from build123d import *

# Parameters (mm, degrees)
SKETCH2_W           = 53.1368
SKETCH2_H           = 28.9814
SKETCH2_W_2         = 5.3848
SKETCH2_H_2         = 3.1242
BOSS_EXTRUDE1_DEPTH = 12.3952
SKETCH3_R           = 4.4831
BOSS_EXTRUDE2_DEPTH = 33.4772
SKETCH5_W           = 3.937
SKETCH5_H           = 3.937
BOSS_EXTRUDE3_DEPTH = 3.048


with BuildPart() as part:
    # Sketch2 → Boss-Extrude1 (new body)
    with BuildSketch(Plane(origin=(0, 0, 0), x_dir=(1, 0, 0), z_dir=(0, 1, 0))):
        Rectangle(SKETCH2_W, SKETCH2_H)
        Polygon((26.5684, -14.4907), (25.2984, -14.4907), (25.2984, -17.6149), (26.5684, -16.3449), align=None)
        with Locations((22.606, -16.0528)):
            Rectangle(SKETCH2_W_2, SKETCH2_H_2)
        Polygon((19.9136, -14.4907), (16.7894, -14.4907), (19.9136, -17.6149), align=None)
        Polygon((-26.5684, -16.3449), (-25.2984, -17.6149), (-25.2984, -14.4907), (-26.5684, -14.4907), align=None)
        with Locations((-22.606, -16.0528)):
            Rectangle(SKETCH2_W_2, SKETCH2_H_2)
        Polygon((-19.9136, -14.4907), (-19.9136, -17.6149), (-16.7894, -14.4907), align=None)
    extrude(amount=BOSS_EXTRUDE1_DEPTH)

    # Sketch3 → Boss-Extrude2 (add)
    with BuildSketch(Plane(origin=(0, 0, -14.4907), x_dir=(-1, 0, 0), z_dir=(0, 0, -1))):
        with Locations(Location((18.6309, 7.9121, 0), (0, 0, 90))):
            Circle(SKETCH3_R)
    extrude(amount=BOSS_EXTRUDE2_DEPTH)

    # Sketch5 → Boss-Extrude3 (add)
    with BuildSketch(Plane(origin=(0, 12.3952, 0), x_dir=(1, 0, 0), z_dir=(0, 1, 0))):
        with Locations((-8.3185, 8.6106)):
            Rectangle(SKETCH5_W, SKETCH5_H)
    extrude(amount=BOSS_EXTRUDE3_DEPTH)


solid = part.part
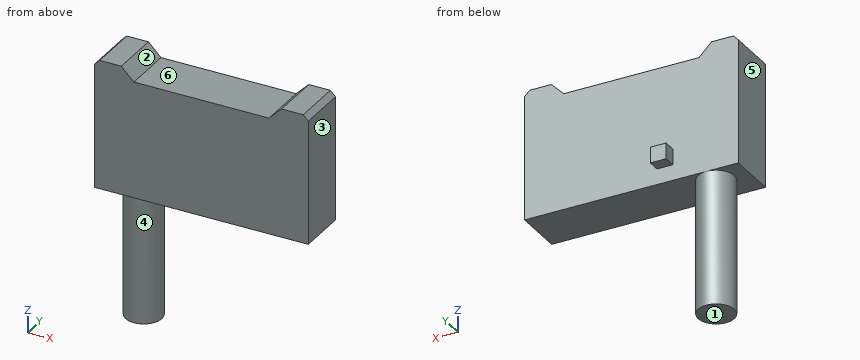
Check sheet for the modelled part. Datum: model origin and axes. Units: mm. Face numbers are marked on the shaded views. A direction names the side the tool comes from. Give positions to 0.01 mm unless a question says otherwise; leave off trailing zeros. Loops run counter-clockwise (first coordinate to the right, second up) from the corner with the lowest first, then second, coordinate; pieces in that order, holes last. Notation, with made-up numbers: M 87.25,-16.5 L 97.25,-16.5 A13 ccw 97.25,-10.5 Z; hole C 5.5,11 d8. An arc over 180 degrees is marked long. Use a Markdown table: item, result. Add a question column.
Q1. Tool access check on the marked faces 5 and 6. Record the directions out of +Z, -Z, +X, -X, +Y, -Y that give a thin tool (end or side, any length) a straight path to the whole face; none if there is none.
Q2. Sectioned sample at D-D, the plane x = 7. Record the cut outline in (y, z).
Q3. Sectioned sample at B-B, the plane x = -15.5. Record the cut outline in (y, z), then the cut area to 3 significant figures.
Q4. Sectioned sample at A-A, the plane y = 7.5. Record the cut outline in (x, z), then the cut area to 3 significant figures.
Q5. Scan lines: line 1 along X through (y, z) = (13, -8.5); line 2 along Z through (x, y) = (10.5, 10.25); line 3 along Z through (x, y) = (-9.5, 14.25). Record each from-to range of solid material in increasing order. Write a range as [from, to].
Q6. Mould release check, pull along X, two halves, no side actions. Record for the marked faces 1, 2, 3 and 4: pulls with the +X half, pulls with the -X half, needs draft (parallel to the pull), parting line crosses it, or undercut.
Q7. Go/stop test with flat-tipped pins: pin 1 (3.5 mm diameter, centred on x = -9, y = 13.5, fed in from +Z); pin 2 (0.9 mm diameter, centred on y = 14, z = -8, fed in from -X); pin 3 (6 mm diameter, centred on x = -11, y = 6.5, fed in from -Z). Record where each tip stops, or that it passes through.
Q8. Sectioned sample at C-C, the plane z = 0.5. Record the cut outline in (x, y), then the cut area to 3 significant figures.
Verdict:
| question | item | result |
|---|---|---|
| 1 | face 5 | +Z, -Z, -X, +Y, -Y |
| 1 | face 6 | +Z, +Y, -Y |
| 2 | outline | M 0,-14.49 L 12.4,-14.49 L 12.4,14.49 L 0,14.49 Z |
| 3 | outline | M 0,-14.49 L 4.7,-14.49 L 4.7,-47.97 L 11.12,-47.97 L 11.12,-14.49 L 12.4,-14.49 L 12.4,14.49 L 0,14.49 Z |
| 3 | area | 574 mm^2 |
| 4 | outline | M -26.57,-14.49 L -23.1,-14.49 L -23.1,-47.97 L -14.17,-47.97 L -14.17,-14.49 L 26.57,-14.49 L 26.57,16.34 L 25.3,17.61 L 19.91,17.61 L 16.79,14.49 L -16.79,14.49 L -19.91,17.61 L -25.3,17.61 L -26.57,16.34 Z |
| 4 | area | 1,890 mm^2 |
| 5 | line 1 | [-10.29, -6.35] |
| 5 | line 2 | [-14.49, 14.49] |
| 5 | line 3 | [-10.58, -6.64] |
| 6 | face 1 | needs draft |
| 6 | face 2 | undercut |
| 6 | face 3 | pulls with the +X half |
| 6 | face 4 | parting line crosses it |
| 7 | pin 1 | z = 14.49 |
| 7 | pin 2 | x = -10.29 |
| 7 | pin 3 | z = -14.49 |
| 8 | outline | M -26.57,0 L 26.57,0 L 26.57,12.4 L -26.57,12.4 Z |
| 8 | area | 659 mm^2 |
